Part print with two shaded views. Sizes in mm from the minimum x, y, z corner. Give positions to 0.01 mm unless a question says otherwise; leave off trailing zeros. Write each loop counter-clockwise with the first axis right and the second up, starting at its lowest first coordinate (ties: lowest second). Pieces come first, ordered by that corner, then holes. Notation, with made-up numbers: (77.25, -37.5) - (94.25, -37.5) arc R18 ccw to (94.25, -15.5) - close; hole circle Ø4 at (17, 64). An arc over 180 degrees is marked (long way). One line per item, written item: value. Start each with the question number.
(1) Cut at B-B, the plane x = 26.9. List the corners of the cut face in (y, z).
(2) Cut at A-A, the plane y = 1.5. List the corners of the cut face in (x, z).
(3) Cut at D-D, the plane x = 5. List the corners of the cut face in (y, z), and give its area (3 significant figures).
(4) Cut at C-C, the plane z = 0.5. List the corners of the cut face in (x, y), and give its area (3 significant figures).
(5) Drop flat-ended pins along their axis: P1, Ø0.6, axis at x = 27, y = 2, coming from the -Z side; P2, Ø1, axis at x = 26.5, z = 2, coming from the -Y side; P3, Ø1.2, axis at x = 26.9, y = 1.5, coming from the -Z side. Give the stop position or say it passes through.
(6) Probe L1, parallel to Y at x = 26.9, z = 1.95; L2, parallel to Y at x = 26.9, z = 1.15; L3, parallel to Y at x = 48.5, z = 0.2. List the from-to ranges inside material, lowest first.
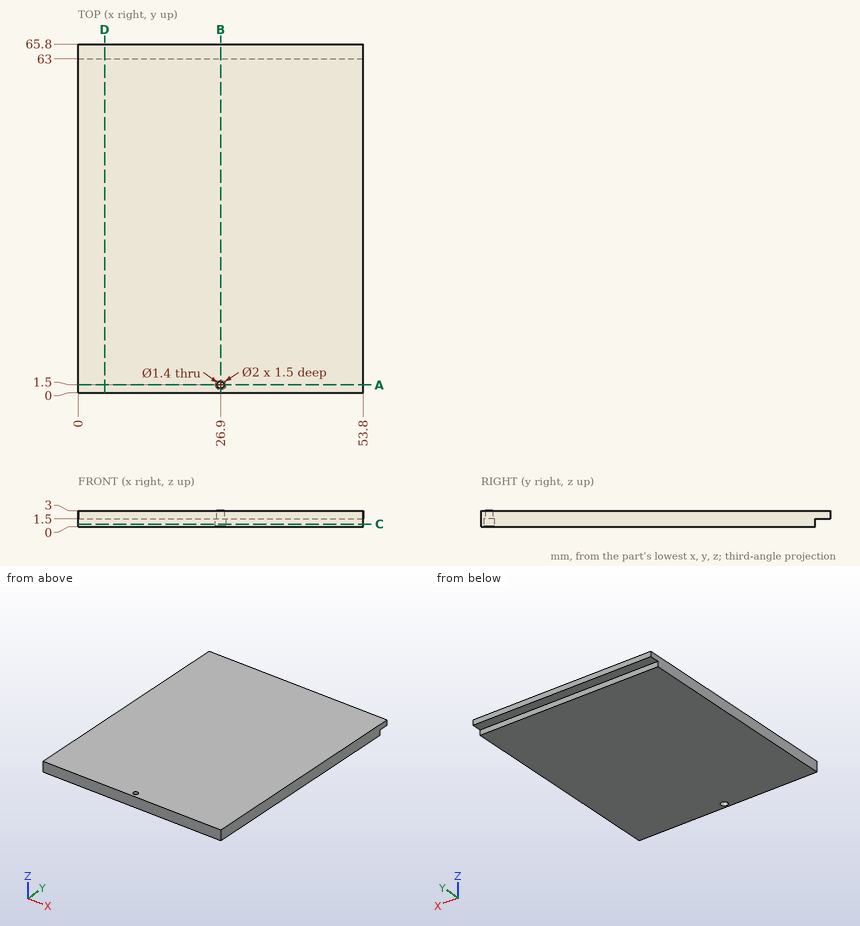
Answers follow:
1. outline: (0, 0) - (0.5, 0) - (0.5, 1.5) - (0.8, 1.5) - (0.8, 3) - (0, 3) - close; (2.2, 1.5) - (2.5, 1.5) - (2.5, 0) - (63, 0) - (63, 1.5) - (65.8, 1.5) - (65.8, 3) - (2.2, 3) - close
2. outline: (0, 0) - (25.9, 0) - (25.9, 1.5) - (26.2, 1.5) - (26.2, 3) - (0, 3) - close; (27.6, 1.5) - (27.9, 1.5) - (27.9, 0) - (53.8, 0) - (53.8, 3) - (27.6, 3) - close
3. outline: (0, 0) - (63, 0) - (63, 1.5) - (65.8, 1.5) - (65.8, 3) - (0, 3) - close
3. area: 193 mm²
4. outline: (0, 0) - (53.8, 0) - (53.8, 63) - (0, 63) - close; hole circle Ø2 at (26.9, 1.5)
4. area: 3,390 mm²
5. P1: stops at z = 1.5
5. P2: stops at y = 0
5. P3: passes through
6. L1: y = 0 to 0.8, 2.2 to 65.8
6. L2: y = 0 to 0.5, 2.5 to 63
6. L3: y = 0 to 63
